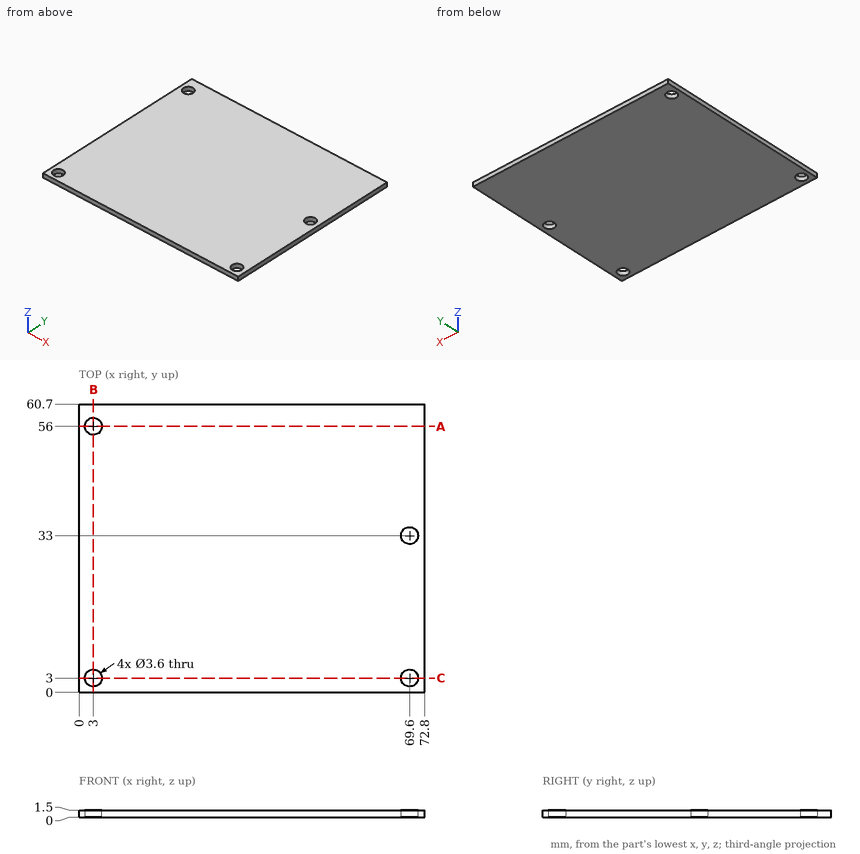
The figure shows three views and two pictorial views of one solid part (mm, origin at its lowest corner). Answer the questions. Give positions to 0.01 mm unless a question says otherwise; leave off trailing zeros. Write each loop counter-clockwise with the first axis right and the second up, starting at its lowest first coordinate (ties: lowest second). Pieces come first, ordered by that corner, then holes. Notation, with made-up numbers: (-13.5, 77) -> (39.5, 77) arc R13 cw to (39.5, 101) -> close; hole circle Ø2 at (-32, 67). An arc over 180 degrees is marked (long way). Answer as a JSON object with one key per item and string values.
1) Section B-B on x = 3 is taken. Write down the section's boundary in (y, z), then the cut area to 4 significant figures.
Findings below:
{"outline": "(0, 0) -> (1.2, 0) -> (1.2, 1.5) -> (0, 1.5) -> close; (4.8, 0) -> (54.2, 0) -> (54.2, 1.5) -> (4.8, 1.5) -> close; (57.8, 0) -> (60.7, 0) -> (60.7, 1.5) -> (57.8, 1.5) -> close", "area": "80.25 mm^2"}
2) Section A-A on y = 56 is taken. Write down the section's boundary in (x, z), then the cut area to 3 significant figures.
Findings below:
{"outline": "(0, 0) -> (1.2, 0) -> (1.2, 1.5) -> (0, 1.5) -> close; (4.8, 0) -> (72.8, 0) -> (72.8, 1.5) -> (4.8, 1.5) -> close", "area": "104 mm^2"}
3) Straight lines are drawn through the part: probe 1 along Y at (x, z) = (3, 0.6); probe 2 along Y at (x, z) = (69.6, 0.8); probe 3 along X at (y, z) = (3, 0.4). For each, find the intervals that lie inside material, in ascending order. Write a range as from..to.
Findings below:
{"probe 1": "y = 0..1.2, 4.8..54.2, 57.8..60.7", "probe 2": "y = 0..1.2, 4.8..31.2, 34.8..60.7", "probe 3": "x = 0..1.2, 4.8..67.8, 71.4..72.8"}
4) Section C-C on y = 3 is taken. Write down the section's boundary in (x, z).
Findings below:
{"outline": "(0, 0) -> (1.2, 0) -> (1.2, 1.5) -> (0, 1.5) -> close; (4.8, 0) -> (67.8, 0) -> (67.8, 1.5) -> (4.8, 1.5) -> close; (71.4, 0) -> (72.8, 0) -> (72.8, 1.5) -> (71.4, 1.5) -> close"}
